Source: three-view drawing plus pictorial views. Frame: mm from the lowest corner of the part. Give positions to 0.01 mm unless a question says otherwise; leave off trailing zeros. Order: outer loops, then holes, each group sorted by start corner. A loop starts at its lowest first (then second) coordinate and runs counter-clockwise, first axis right, second up.
1) Section B-B, the plane z = 82. Return loops of the section in (x, y) (1 decimal).
2) Section D-D, the plane y = 2.65. Give the number of separate pieces and of enclosed holes in the cut face.
3) Material intervals for line 1 (X direction, y = 3.15, z = 12.75); line 2 (Z direction, x = 48.5, y = 1.3); line 3 (X direction, y = 1.25, z = 46.5) (1 decimal), sorted ascending.
4) Section C-C, the plane x = 12.75. Return loops of the section in (y, z).
5) Section A-A, the plane z = 49. Return loops of the section in (x, y) (1 decimal).
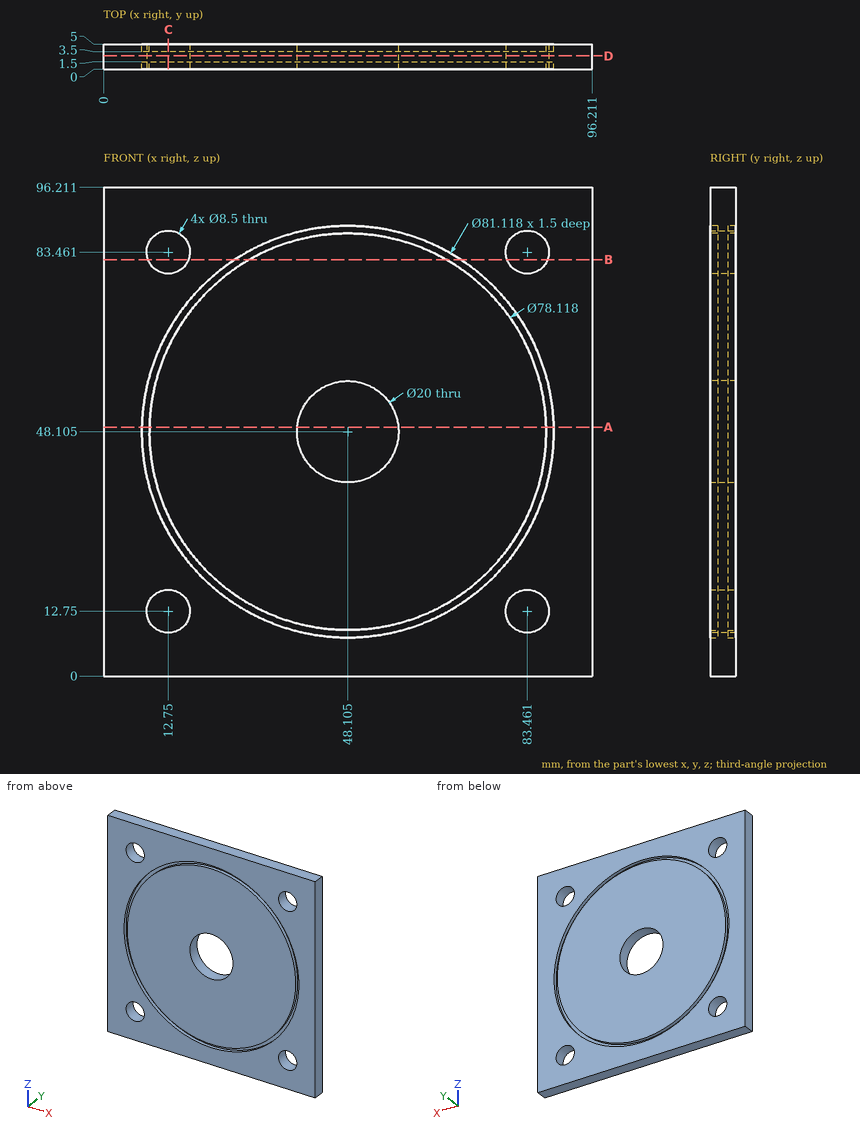
From the geometry:
1. outline: (0, 0) - (8.8, 0) - (8.8, 5) - (0, 5) - close; (16.7, 0) - (25.8, 0) - (25.8, 1.5) - (28.7, 1.5) - (28.7, 0) - (67.5, 0) - (67.5, 1.5) - (70.4, 1.5) - (70.4, 0) - (79.5, 0) - (79.5, 5) - (70.4, 5) - (70.4, 3.5) - (67.5, 3.5) - (67.5, 5) - (28.7, 5) - (28.7, 3.5) - (25.8, 3.5) - (25.8, 5) - (16.7, 5) - close; (87.5, 0) - (96.2, 0) - (96.2, 5) - (87.5, 5) - close
2. separate pieces: 1
2. enclosed holes: 5
3. line 1: x = 0 to 8.5, 17 to 79.21, 87.71 to 96.21
3. line 2: z = 0 to 7.55, 9.05 to 38.11, 58.1 to 87.16, 88.66 to 96.21
3. line 3: x = 0 to 7.6, 9.1 to 38.2, 58 to 87.1, 88.6 to 96.2
4. outline: (0, 0) - (5, 0) - (5, 8.5) - (0, 8.5) - close; (0, 17) - (5, 17) - (5, 28.23) - (3.5, 28.23) - (3.5, 31.5) - (5, 31.5) - (5, 64.71) - (3.5, 64.71) - (3.5, 67.98) - (5, 67.98) - (5, 79.21) - (0, 79.21) - (0, 67.98) - (1.5, 67.98) - (1.5, 64.71) - (0, 64.71) - (0, 31.5) - (1.5, 31.5) - (1.5, 28.23) - (0, 28.23) - close; (0, 87.71) - (5, 87.71) - (5, 96.21) - (0, 96.21) - close
5. outline: (0, 0) - (7.6, 0) - (7.6, 1.5) - (9.1, 1.5) - (9.1, 0) - (38.1, 0) - (38.1, 5) - (9.1, 5) - (9.1, 3.5) - (7.6, 3.5) - (7.6, 5) - (0, 5) - close; (58.1, 0) - (87.2, 0) - (87.2, 1.5) - (88.7, 1.5) - (88.7, 0) - (96.2, 0) - (96.2, 5) - (88.7, 5) - (88.7, 3.5) - (87.2, 3.5) - (87.2, 5) - (58.1, 5) - close
